Model file for the job. Use its own axes, mm. Face numbers are marked on the shaded views. A direction names the side the tool comes from. Give positions to 0.01 mm unless a question says otherwise; leave off trailing zeros. Loops run counter-clockwise (first coordinate to the right, second up) from the corner with the lowest first, then second, coordinate; pieces in that order, holes last. Notation, with made-up numbers: (58, 68.5) - (93, 68.5) arc R28 cw to (93, 102.5) - close; hole circle Ø2 at (-22.5, 52.5). An arc over 180 degrees is marked (long way). Use a Markdown table: item, result.
Solid Edge part; units mm, degrees
sketch "Sketch1" plane through (0, 0, 0) normal (0, 0, 1) x (1, 0, 0)
  line L0 (-102.6529, 0) -> (-51.3264, -88.9)
  line L1 (-51.3264, -88.9) -> (51.3264, -88.9)
  line L2 (51.3264, -88.9) -> (102.6529, 0)
  line L3 (102.6529, 0) -> (51.3264, 88.9)
  line L4 (51.3264, 88.9) -> (-51.3264, 88.9)
  line L5 (-51.3264, 88.9) -> (-102.6529, 0)
extrude "Protrusion1" add sketch "Sketch1" along normal blind 63.5
sketch "Sketch2" plane through (0, 0, 0) normal (0, 0, -1) x (-0.5, 0.866, 0)
  circle A0 centre (0, 0) radius 63.5
extrude "ExtrudedProtrusion_2" add sketch "Sketch2" along normal blind 254
sketch "Sketch3" plane through (0, 0, 0) normal (0, 0, -1) x (0.5, 0.866, 0)
  circle A0 centre (0, 0) radius 127
extrude "ExtrudedProtrusion_3" add sketch "Sketch3" along normal blind 12.7
sketch "Sketch4" plane through (0, 0, 0) normal (0, -1, 0) x (1, 0, 0)
  line L0 (88.9, 63.5) -> (126.295, 41.91)
revolve "RevolvedCutout1" cut sketch "Sketch4" angle 360 about axis through (0, 0, 0) along (0, 0, 1) material side at (107.6225, 0, 52.7483)
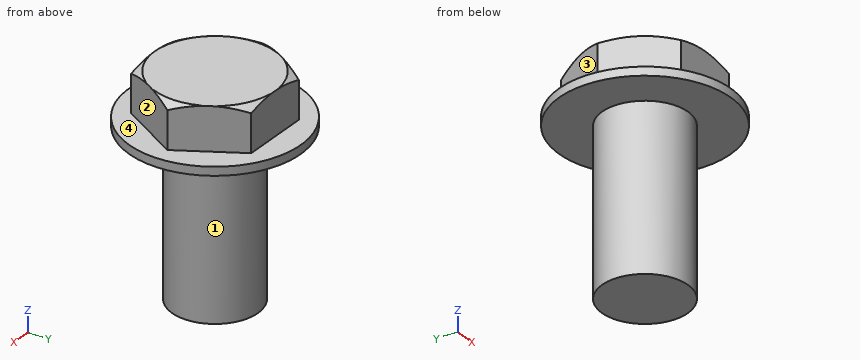
(1) Slice it at A-A, the plane z = -8.5. Write the cut outline in (x, y).
Computed:
| item | result |
|---|---|
| outline | circle Ø254 at (0, 0) |
(2) Drill centre lines: probe 1 along Z at (x, y) = (-8, -105); probe 2 along X at (y, z) = (-1, -125.5); probe 3 along Y at (x, z) = (-1.5, -158.5). Where is each one in solid material? Low to high. Write a range as [from, to].
Computed:
| item | result |
|---|---|
| probe 1 | [-12.7, 0] |
| probe 2 | [-63.49, 63.49] |
| probe 3 | [-63.48, 63.48] |
(3) 3-axis set-ups, long thin cutter, end or side, ignore diameter. For the marked faces 1, 2, 3 and 4: which of +Z, -Z, +X, -X, +Y, -Y reach the whole face in a straight line?
Computed:
| item | result |
|---|---|
| face 1 | -Z |
| face 2 | +Z, +X, -Y |
| face 3 | +Z, -X, +Y |
| face 4 | +Z |
(4) Pin check, flat tips, straight feed: P1, Ø10, axis at y = -16.5, z = -118.5, coming from the +X side; P2, Ø10, axis at y = 58.5, z = -59.5, coming from the +X side; P3, Ø3, axis at x = 69, y = 94, coming from the +Z side. Stop position of each tip, or through.
Computed:
| item | result |
|---|---|
| P1 | x = 62.45 |
| P2 | x = 34.21 |
| P3 | z = 0 |
